Input: part model. Units: mm. Frame: model coordinates. A direction names the side the tool comes from. Give positions to 0.01 mm unless a question says otherwise; leave off trailing zeros. Loops run counter-clockwise (first coordinate to the right, second up) from the corner with the lowest first, then second, coordinate; pieces in that order, holes last. Notation, with made-up numbers: (-11, 46) - (-2, 46) arc R28 cw to (-2, 65) - close; hole circle Ø4 at (0.5, 76). An arc over 180 degrees is marked (long way). One line per question, with ' | ' between items. Start each with the question number.
from build123d import *

# Parameters (mm, degrees)
SKETCH1_W           = 95.41
SKETCH1_H           = 184.3
SKETCH1_R           = 16.565
BOSS_EXTRUDE1_DEPTH = 9.43
CHAMFER1_SIZE       = 3
SKETCH2_R           = 36.575
CUT_EXTRUDE1_DEPTH  = 1.34
SKETCH3_R           = 9.525
CUT_EXTRUDE2_DEPTH  = 10.43
SKETCH4_R           = 2.8
CUT_EXTRUDE3_DEPTH  = 10.43
SKETCH5_R           = 4.6
CUT_EXTRUDE4_DEPTH  = 4.72
SKETCH6_R           = 1.98
CUT_EXTRUDE5_DEPTH  = 10.43
SKETCH7_R           = 2.06
CUT_EXTRUDE6_DEPTH  = 6.93
SKETCH9_R           = 0.77
CUT_EXTRUDE7_DEPTH  = 10.43


with BuildPart() as part:
    # Sketch1 → Boss-Extrude1 (new body)
    with BuildSketch(Plane.XY):
        with Locations((47.705, 92.15)):
            Rectangle(SKETCH1_W, SKETCH1_H)
        with Locations((41.365, 136.635)):
            Circle(SKETCH1_R, mode=Mode.SUBTRACT)
        with Locations((41.365, 47.785)):
            Circle(SKETCH1_R, mode=Mode.SUBTRACT)
    extrude(amount=BOSS_EXTRUDE1_DEPTH)

    # Chamfer1
    chamfer1_edges = [part.edges().sort_by_distance(p)[0] for p in [
        (95.41, 184.3, 4.715),
    ]]
    chamfer(chamfer1_edges, length=CHAMFER1_SIZE)

    # Sketch2 → Cut-Extrude1 (cut)
    with BuildSketch(Plane.XY.offset(9.43)):
        with Locations((41.365, 136.635)):
            Circle(SKETCH2_R)
        with Locations((41.365, 47.785)):
            Circle(SKETCH2_R)
    extrude(amount=-CUT_EXTRUDE1_DEPTH, mode=Mode.SUBTRACT)

    # Sketch3 → Cut-Extrude2 (cut, through all)
    with BuildSketch(Plane.XY.offset(9.43)):
        with Locations((41.365, 98.535)):
            Circle(SKETCH3_R)
    extrude(amount=-CUT_EXTRUDE2_DEPTH, mode=Mode.SUBTRACT)

    # Sketch4 → Cut-Extrude3 (cut, through all)
    with BuildSketch(Plane.XY.offset(9.43)):
        with Locations((19.23, 179.5)):
            Circle(SKETCH4_R)
        with Locations((57.29, 179.5)):
            Circle(SKETCH4_R)
        with Locations((19.23, 6.44)):
            Circle(SKETCH4_R)
        with Locations((57.29, 6.44)):
            Circle(SKETCH4_R)
    extrude(amount=-CUT_EXTRUDE3_DEPTH, mode=Mode.SUBTRACT)

    # Sketch5 → Cut-Extrude4 (cut)
    with BuildSketch(Plane.XY.offset(9.43)):
        with Locations((19.23, 179.5)):
            Circle(SKETCH5_R)
        with Locations((57.29, 179.5)):
            Circle(SKETCH5_R)
        with Locations((19.23, 6.44)):
            Circle(SKETCH5_R)
        with Locations((57.29, 6.44)):
            Circle(SKETCH5_R)
    extrude(amount=-CUT_EXTRUDE4_DEPTH, mode=Mode.SUBTRACT)

    # Sketch6 → Cut-Extrude5 (cut, through all)
    with BuildSketch(Plane.XY.offset(9.43)):
        with Locations((6.567, 171.433)):
            Circle(SKETCH6_R)
        with Locations((76.163, 171.433)):
            Circle(SKETCH6_R)
        with Locations((76.163, 101.837)):
            Circle(SKETCH6_R)
        with Locations((6.567, 101.837)):
            Circle(SKETCH6_R)
        with Locations((6.567, 82.583)):
            Circle(SKETCH6_R)
        with Locations((76.163, 82.583)):
            Circle(SKETCH6_R)
        with Locations((76.163, 12.987)):
            Circle(SKETCH6_R)
        with Locations((6.567, 12.987)):
            Circle(SKETCH6_R)
    extrude(amount=-CUT_EXTRUDE5_DEPTH, mode=Mode.SUBTRACT)

    # Sketch7 → Cut-Extrude6 (cut)
    with BuildSketch(Plane(origin=(95.41, 0, 0), x_dir=(0, 0, -1), z_dir=(1, 0, 0))):
        with Locations((-4.715, 175.02)):
            Circle(SKETCH7_R)
        with Locations((-4.715, 9.6)):
            Circle(SKETCH7_R)
    extrude(amount=-CUT_EXTRUDE6_DEPTH, mode=Mode.SUBTRACT)

    # Sketch9 → Cut-Extrude7 (cut, through all)
    with BuildSketch(Plane(origin=(0, 0, 0), x_dir=(-1, 0, 0), z_dir=(0, 0, -1))):
        with Locations((-89.08, 162.035)):
            Circle(SKETCH9_R)
        with Locations((-63.68, 162.035)):
            Circle(SKETCH9_R)
        with Locations((-89.08, 136.635)):
            Circle(SKETCH9_R)
        with Locations((-63.68, 136.635)):
            Circle(SKETCH9_R)
        with Locations((-89.08, 73.185)):
            Circle(SKETCH9_R)
        with Locations((-63.68, 73.185)):
            Circle(SKETCH9_R)
        with Locations((-89.08, 47.785)):
            Circle(SKETCH9_R)
        with Locations((-63.68, 47.785)):
            Circle(SKETCH9_R)
    extrude(amount=-CUT_EXTRUDE7_DEPTH, mode=Mode.SUBTRACT)


solid = part.part
Q1. Section C-C, the plane x = 42.5. Output: boundary loops of the cut face in (y, z).
Q2. Access query for faces 5 (the face through (6.309, 84.546, 4.781)), 6 (the face through (15.84, 9.55, 7.1)). Directions: +Z, -Z, +X, -X, +Y, -Y. A direction counts if a zero-diameter tool reaches every point of the face in a straight line with its end or side. Return the directions, or none.
Q3. First-contact query: pin 1 (7.5 mm diameter, centred on x = 57.29, y = 6.44, fed in from +Z); pin 2 (3.5 mm diameter, centred on x = 57.29, y = 179.5, fed in from +Z); pin 3 (2.5 mm diameter, centred on x = 63.68, y = 162.035, fed in from +Z); pin 4 (2 mm diameter, centred on y = 10.5, z = 4.5, fed in from +X). Flat tips, straight axial feed; report the tip coordinate or a pass-through.
Q4. Section A-A, the plane y = 179.5. Output: boundary loops of the cut face in (x, z).
Q5. Section D-D, the plane y = 33. Output: boundary loops of the cut face in (x, z), plus the area to 3 significant figures.
Q6. Line query: L1, parallel to Y at x = 63.68, z = 2 (3 decimals); L2, parallel to X at y = 47.5, z = 2.75; L3, parallel to Y at x = 75, z = 5.25. Output: solid intervals per line, ascending. Write a range as from..to.
Q7. Section B-B, the plane x = 6.5. Output: boundary loops of the cut face in (y, z).
Q8. Draft query along Z for faces 1 (the face through (91.99, 7.59, 5.16)), 2 (the face through (88.48, 175, 5)), 3 (the face through (17.008, 4.736, 2.388)), 4 (the face through (22.2, 179.6, 4.71)). Return one class per face: +Z half, -Z half, draft (parallel to the pull), parting line (faces both ways), or undercut.
Solved:
1) outline: (0, 0) - (31.26, 0) - (31.26, 8.09) - (11.23, 8.09) - (11.23, 9.43) - (0, 9.43) - close; (64.31, 0) - (89.08, 0) - (89.08, 9.43) - (84.34, 9.43) - (84.34, 8.09) - (64.31, 8.09) - close; (107.99, 0) - (120.11, 0) - (120.11, 8.09) - (107.99, 8.09) - close; (153.16, 0) - (184.3, 0) - (184.3, 9.43) - (173.19, 9.43) - (173.19, 8.09) - (153.16, 8.09) - close
2) face 5: +Z, -Z | face 6: +Z
3) pin 1: stops at z = 4.71 | pin 2: passes through | pin 3: stops at z = 8.09 | pin 4: stops at x = 88.48
4) outline: (0, 0) - (16.43, 0) - (16.43, 4.71) - (14.63, 4.71) - (14.63, 9.43) - (0, 9.43) - close; (22.03, 0) - (54.49, 0) - (54.49, 4.71) - (52.69, 4.71) - (52.69, 9.43) - (23.83, 9.43) - (23.83, 4.71) - (22.03, 4.71) - close; (60.09, 0) - (95.41, 0) - (95.41, 9.43) - (61.89, 9.43) - (61.89, 4.71) - (60.09, 4.71) - close
5) outline: (0, 0) - (33.89, 0) - (33.89, 8.09) - (7.91, 8.09) - (7.91, 9.43) - (0, 9.43) - close; (48.84, 0) - (95.41, 0) - (95.41, 9.43) - (74.82, 9.43) - (74.82, 8.09) - (48.84, 8.09) - close | area: 689 mm²
6) L1: y = 0..47.015, 48.555..72.415, 73.955..135.865, 137.405..161.265, 162.805..184.3 | L2: x = 0..24.8, 57.93..62.96, 64.4..88.36, 89.8..95.41 | L3: y = 0..11.38, 14.59..80.98, 84.19..100.23, 103.44..169.83, 173.04..184.3
7) outline: (0, 0) - (11.01, 0) - (11.01, 9.43) - (0, 9.43) - close; (14.97, 0) - (80.6, 0) - (80.6, 9.43) - (58.84, 9.43) - (58.84, 8.09) - (36.73, 8.09) - (36.73, 9.43) - (14.97, 9.43) - close; (84.56, 0) - (99.86, 0) - (99.86, 9.43) - (84.56, 9.43) - close; (103.82, 0) - (169.45, 0) - (169.45, 9.43) - (147.69, 9.43) - (147.69, 8.09) - (125.58, 8.09) - (125.58, 9.43) - (103.82, 9.43) - close; (173.41, 0) - (184.3, 0) - (184.3, 9.43) - (173.41, 9.43) - close
8) face 1: undercut | face 2: undercut | face 3: draft | face 4: +Z half
